```python
from build123d import *

# Parameters (mm, degrees)
SKETCH_1_R      = 70
EXTRUDE_1_DEPTH = 3


with BuildPart() as part:
    # Эскиз1 → Бобышка-Вытянуть1 (new body)
    with BuildSketch(Plane(origin=(0, 0, 0), x_dir=(1, 0, 0), z_dir=(0, 1, 0))):
        with Locations(Location((0, 0, 0), (0, 0, 270))):
            Circle(SKETCH_1_R)
        with BuildLine():
            ThreePointArc((-5.991828083, 57.186956522), (-22.004297361, 53.123073119), (-36.200422482, 44.674147021))
            ThreePointArc((-36.200422482, 44.674147021), (-44.901280605, 44.901280605), (-44.674147021, 36.200422482))
            ThreePointArc((-44.674147021, 36.200422482), (-53.123073119, 22.004297361), (-57.186956522, 5.991828083))
            ThreePointArc((-57.186956522, 5.991828083), (-63.5, 0), (-57.186956522, -5.991828083))
            ThreePointArc((-57.186956522, -5.991828083), (-53.123073119, -22.004297361), (-44.674147021, -36.200422482))
            ThreePointArc((-44.674147021, -36.200422482), (-44.901280605, -44.901280605), (-36.200422482, -44.674147021))
            ThreePointArc((-36.200422482, -44.674147021), (-22.004297361, -53.123073119), (-5.991828083, -57.186956522))
            ThreePointArc((-5.991828083, -57.186956522), (0, -63.5), (5.991828083, -57.186956522))
            ThreePointArc((5.991828083, -57.186956522), (22.004297361, -53.123073119), (36.200422482, -44.674147021))
            ThreePointArc((36.200422482, -44.674147021), (44.901280605, -44.901280605), (44.674147021, -36.200422482))
            ThreePointArc((44.674147021, -36.200422482), (53.123073119, -22.004297361), (57.186956522, -5.991828083))
            ThreePointArc((57.186956522, -5.991828083), (63.5, 0), (57.186956522, 5.991828083))
            ThreePointArc((57.186956522, 5.991828083), (53.123073119, 22.004297361), (44.674147021, 36.200422482))
            ThreePointArc((44.674147021, 36.200422482), (44.901280605, 44.901280605), (36.200422482, 44.674147021))
            ThreePointArc((36.200422482, 44.674147021), (22.004297361, 53.123073119), (5.991828083, 57.186956522))
            ThreePointArc((5.991828083, 57.186956522), (0, 63.5), (-5.991828083, 57.186956522))
        make_face(mode=Mode.SUBTRACT)
    extrude(amount=EXTRUDE_1_DEPTH)


solid = part.part
```
Input: part model. Units: mm. Frame: model coordinates. A direction names the side the tool comes from. Give positions to 0.01 mm unless a question says otherwise; leave off trailing zeros. Write each loop counter-clockwise with the first axis right and the second up, starting at its lowest first coordinate (ties: lowest second). Pieces come first, ordered by that corner, then holes. Notation, with made-up numbers: (43, 70) - (53, 70) arc R9 ccw to (53, 76) - close; hole circle Ø7 at (56, 44.5). An arc over 180 degrees is marked (long way). Write item = value, one per line. Start each with the question number.
1. Section query A-A, the plane x = 0. Output: boundary loops of the cut face in (y, z).
2. First-contact query: pin 1 Ø1.5 at (x, y) = (31, 2.5) entering from -Z. Flat tip, straight axial feed; report the tip coordinate or a pass-through.
3. Access query for faces 1 (the flat face through (-57, 3, 10)), 2 (the cylindrical face through (-63.5, 1.5, -0.1)). Directions: +Z, -Z, +X, -X, +Y, -Y. A direction counts if a zero-diameter tool reaches every point of the face in a straight line with its end or side. Return the directions, or none.
4. Section query C-C, the plane y = 1.95. Output: boundary loops of the cut face in (x, z), then the cut area to 3 significant figures.
5. Ray query, L1, parallel to Z at x = -17, y = 2.55; L2, parallel to X at y = 2, z = -26; L3, parallel to Z at x = 4, y = 1.25. Return the intervals inside material, ascending.
6. Mould query, pull axis X, two halves, no side actions, for faces 3 (the cylindrical face through (-42.594, 1.479, -55.55)), 4 (the cylindrical face through (21.79, 1.48, 53.21)), 5 (the flat face through (-57, 0, 10)). Classes: released by +X, released by -X, zero draft, split by the parting line, or undercut.
7. Section query B-B, the plane z = 0. Output: boundary loops of the cut face in (x, y).
Check sheet entries:
q1.outline = (0, -70) - (3, -70) - (3, -63.5) - (0, -63.5) - close; (0, 63.5) - (3, 63.5) - (3, 70) - (0, 70) - close
q2.pin_1 = -63.13
q3.face_1 = +Z, -Z, +X, -X, +Y
q3.face_2 = +Y, -Y
q4.outline = circle Ø140 at (0, 0); hole (-57.19, -5.99) arc R57.5 ccw to (-44.67, -36.2) arc R6 ccw (long way) to (-36.2, -44.67) arc R57.5 ccw to (-5.99, -57.19) arc R6 ccw (long way) to (5.99, -57.19) arc R57.5 ccw to (36.2, -44.67) arc R6 ccw (long way) to (44.67, -36.2) arc R57.5 ccw to (57.19, -5.99) arc R6 ccw (long way) to (57.19, 5.99) arc R57.5 ccw to (44.67, 36.2) arc R6 ccw (long way) to (36.2, 44.67) arc R57.5 ccw to (5.99, 57.19) arc R6 ccw (long way) to (-5.99, 57.19) arc R57.5 ccw to (-36.2, 44.67) arc R6 ccw (long way) to (-44.67, 36.2) arc R57.5 ccw to (-57.19, 5.99) arc R6 ccw (long way) to start
q4.area = 4,540 mm2
q5.L1 = -67.9 to -54.93, 54.93 to 67.9
q5.L2 = -64.99 to -51.29, 51.29 to 64.99
q5.L3 = -69.89 to -61.97, 61.97 to 69.89
q6.face_3 = split by the parting line
q6.face_4 = undercut
q6.face_5 = zero draft
q7.outline = (-70, 0) - (-63.5, 0) - (-63.5, 3) - (-70, 3) - close; (63.5, 0) - (70, 0) - (70, 3) - (63.5, 3) - close
